Read the model definition and answer for the solid it produces. Units are mm, in the model's axes. Face numbers are marked on the shaded views. Give positions to 0.01 mm unless a question says otherwise; leave off trailing zeros. Write each loop counter-clockwise with the first axis right and the second up, starting at its lowest first coordinate (ties: lowest second). Pieces come first, ordered by that corner, then holes.
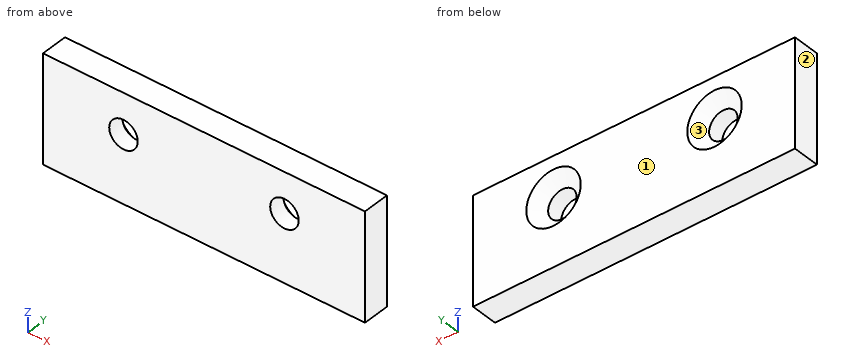
```python
from build123d import *

# Parameters (mm, degrees)
SKETCH1_W                                           = 76.2
SKETCH1_H                                           = 25.4
BOSS_EXTRUDE1_DEPTH                                 = 6.35
CSK_FOR_1_4_FLAT_HEAD_MACHINE_SCREW_100_D           = 6.7564
CSK_FOR_1_4_FLAT_HEAD_MACHINE_SCREW_100_CSINK_D     = 12.8778
CSK_FOR_1_4_FLAT_HEAD_MACHINE_SCREW_100_CSINK_ANGLE = 100


with BuildPart() as part:
    # Sketch1 → Boss-Extrude1 (new body)
    with BuildSketch(Plane(origin=(0, 0, 0), x_dir=(1, 0, 0), z_dir=(0, 1, 0))):
        with Locations((38.1, 12.7)):
            Rectangle(SKETCH1_W, SKETCH1_H)
    extrude(amount=-BOSS_EXTRUDE1_DEPTH)

    # CSK for 1/4 Flat Head Machine Screw (100)1 (through all)
    with Locations(Plane(origin=(0, 0, 0), x_dir=(1, 0, 0), z_dir=(0, 1, 0))):
        with Locations((19.05, 9.525), (57.15, 9.525)):
            CounterSinkHole(CSK_FOR_1_4_FLAT_HEAD_MACHINE_SCREW_100_D / 2, CSK_FOR_1_4_FLAT_HEAD_MACHINE_SCREW_100_CSINK_D / 2, counter_sink_angle=CSK_FOR_1_4_FLAT_HEAD_MACHINE_SCREW_100_CSINK_ANGLE)


solid = part.part
```
Item 1: Determine the mould class of the marked faces 1, 2 and 3 for opening direction X: pulls with the +X half, pulls with the -X half, needs draft (parallel to the pull), parting line crosses it, or undercut.
Result set:
face 1: needs draft
face 2: pulls with the -X half
face 3: undercut
Item 2: Section B-B (y = -1.75) is taken. Write down the section's boundary in (x, z) (3 decimals).
Result set:
outline: (0, -25.4) - (76.2, -25.4) - (76.2, 0) - (0, 0) - close; hole circle Ø8.707 at (19.05, -9.525); hole circle Ø8.707 at (57.15, -9.525)
Item 3: Section D-D (y = -4.75) is taken. Write down the section's boundary in (x, z) (3 decimals).
Result set:
outline: (0, -25.4) - (76.2, -25.4) - (76.2, 0) - (0, 0) - close; hole circle Ø6.756 at (19.05, -9.525); hole circle Ø6.756 at (57.15, -9.525)
Item 4: Section A-A (x = 57.15) is taken. Write down the section's boundary in (y, z), and give its area (3 significant figures).
Result set:
outline: (-6.35, -25.4) - (0, -25.4) - (0, -15.96) - (-2.57, -12.9) - (-6.35, -12.9) - close; (-6.35, -6.15) - (-2.57, -6.15) - (0, -3.09) - (0, 0) - (-6.35, 0) - close
area: 111 mm2
Item 5: Section C-C (z = -10.5) is taken. Give the number of separate pieces and of enclosed holes in the cut face, and give its area (3 significant figures).
Result set:
separate pieces: 3
enclosed holes: 0
area: 386 mm2
Item 6: This flat-tipped pin is pushed along its axis until it touches: pin 1 Ø6 at (x, z) = (57.15, -9.525) entering from -Y. Where does it stop, or does it pass through?
Result set:
pin 1: passes through
Item 7: Find the intervals of material crossed by line 1 along Z through (x, y) = (19.05, -5.2); line 2 along X through (y, z) = (-3.5, -9); line 3 along X through (y, z) = (-5.5, -11), in increasing order.
Result set:
line 1: z = -25.4 to -12.9, -6.15 to 0
line 2: x = 0 to 15.71, 22.39 to 53.81, 60.49 to 76.2
line 3: x = 0 to 16.01, 22.09 to 54.11, 60.19 to 76.2
